```python
from build123d import *

# Parameters (mm, degrees)
ANGLE_DEPTH        = 30
SKETCH2_R          = 1.5
CUT_EXTRUDE1_DEPTH = 50
SKETCH3_R          = 1.5
CUT_EXTRUDE2_DEPTH = 50
SKETCH4_W          = 30
SKETCH4_H          = 3.15
CUT_EXTRUDE3_DEPTH = 50
SKETCH5_W          = 8.4
SKETCH5_H          = 30
CUT_EXTRUDE4_DEPTH = 50


with BuildPart() as part:
    # Sketch1 → Angle (new body)
    with BuildSketch(Plane.XY):
        Polygon((0, 0), (-23.4, 0), (-23.4, 1.6), (1.6, 1.6), (1.6, -23.4), (0, -23.4), align=None)
    extrude(amount=ANGLE_DEPTH)

    # Sketch2 → Cut-Extrude1 (cut)
    with BuildSketch(Plane.XZ):
        with Locations((-7.5, 5)):
            Circle(SKETCH2_R)
        with Locations((-7.5, 25)):
            Circle(SKETCH2_R)
    extrude(amount=-CUT_EXTRUDE1_DEPTH, mode=Mode.SUBTRACT)

    # Sketch3 → Cut-Extrude2 (cut)
    with BuildSketch(Plane.ZY):
        with Locations(Location((4, -7.5, 0), (0, 0, 270))):
            Circle(SKETCH3_R)
        with Locations(Location((26, -7.5, 0), (0, 0, 270))):
            Circle(SKETCH3_R)
        with Locations(Location((4, -17.5, 0), (0, 0, 270))):
            Circle(SKETCH3_R)
        with Locations(Location((26, -17.5, 0), (0, 0, 270))):
            Circle(SKETCH3_R)
    extrude(amount=-CUT_EXTRUDE2_DEPTH, mode=Mode.SUBTRACT)

    # Sketch4 → Cut-Extrude3 (cut)
    with BuildSketch(Plane.ZY):
        with Locations((15, -21.825)):
            Rectangle(SKETCH4_W, SKETCH4_H)
    extrude(amount=-CUT_EXTRUDE3_DEPTH, mode=Mode.SUBTRACT)

    # Sketch5 → Cut-Extrude4 (cut)
    with BuildSketch(Plane.XZ):
        with Locations((-19.2, 15)):
            Rectangle(SKETCH5_W, SKETCH5_H)
    extrude(amount=-CUT_EXTRUDE4_DEPTH, mode=Mode.SUBTRACT)


solid = part.part
```
The model under review builds one solid part; all positions refer to its coordinate system, in mm. A direction names the side the tool comes from. Round coordinates to 2 decimals unless told otherwise and drop trailing zeros. Write each loop counter-clockwise with the first axis right and the second up, starting at its lowest first coordinate (ties: lowest second). Pieces come first, ordered by that corner, then holes.
(1) We need section B-B on x = -7.5. Give the boundary of the cut face in (y, z), and give its area (3 significant figures).
(2) We need section A-A on y = -7.5. Give the boundary of the cut face in (x, z).
(3) We need section C-C on z = 25. Give the boundary of the cut face in (x, y).
(4) Insertion check: pin 1 (6 mm diameter, centred on y = -17, z = 20.5, fed in from -X); pin 2 (2 mm diameter, centred on y = -6.5, z = 5, fed in from +X); pin 3 (1.8 mm diameter, centred on y = -17.5, z = 4, fed in from -X); pin 4 (6 mm diameter, centred on x = -5.5, z = 19.5, fed in from -Y). Each pin has a flat end and moves straight along its axis. Give the tip position at first contact, or say it passes through.
(5) Machinability: for faces 4 (the flat face through (1.6, -9, 15)), 5 (the flat face through (-7, 0, 15)), which of the approach directions +Z, -Z, +X, -X, +Y, -Y give a long, thin tool a straight path to every point of the face, cutting with its end or side? Answer none if there is none.
(6) We need section D-D on z = 9.75. Give the boundary of the cut face in (x, y), and give its area (3 significant figures).
(7) Wall thickness on L1, parallel to Z at x = -7.5, y = 0.55; L2, parallel to Z at x = 0.4, y = -7.5; L3, parallel to Y at x = -3.5, z = 4: over which ranges is each line inside the solid? List them lowest first.
(8) Mouldability with a two-part tool opening along Z and no side actions: class faces 1 (the flat face through (1, -6, 0)), 2 (the flat face through (-15, 1, 15)), 3 (the cylindrical face through (0.79, -16.39, 27.01)) as +Z half, -Z half, draft (parallel to the pull), parting line (faces both ways), or undercut.
Findings below:
1. outline: (0, 0) - (1.6, 0) - (1.6, 3.5) - (0, 3.5) - close; (0, 6.5) - (1.6, 6.5) - (1.6, 23.5) - (0, 23.5) - close; (0, 26.5) - (1.6, 26.5) - (1.6, 30) - (0, 30) - close
1. area: 38.4 mm2
2. outline: (0, 0) - (1.6, 0) - (1.6, 2.5) - (0, 2.5) - close; (0, 5.5) - (1.6, 5.5) - (1.6, 24.5) - (0, 24.5) - close; (0, 27.5) - (1.6, 27.5) - (1.6, 30) - (0, 30) - close
3. outline: (-15, 0) - (-9, 0) - (-9, 1.6) - (-15, 1.6) - close; (-6, 0) - (0, 0) - (0, -6.38) - (1.6, -6.38) - (1.6, 1.6) - (-6, 1.6) - close; (0, -20.25) - (1.6, -20.25) - (1.6, -18.62) - (0, -18.62) - close; (0, -16.38) - (1.6, -16.38) - (1.6, -8.62) - (0, -8.62) - close
4. pin 1: stops at x = 0
4. pin 2: stops at x = 1.6
4. pin 3: passes through
4. pin 4: stops at y = 0
5. face 4: +Z, -Z, +X, +Y, -Y
5. face 5: +Z, -Z, -X, -Y
6. outline: (-15, 0) - (0, 0) - (0, -20.25) - (1.6, -20.25) - (1.6, 1.6) - (-15, 1.6) - close
6. area: 59.0 mm2
7. L1: z = 0 to 3.5, 6.5 to 23.5, 26.5 to 30
7. L2: z = 0 to 2.5, 5.5 to 24.5, 27.5 to 30
7. L3: y = 0 to 1.6
8. face 1: -Z half
8. face 2: draft
8. face 3: undercut
